Design review of the part built by this model. Coordinates are the model's own, in mm. A direction names the side the tool comes from. Coordinates: 2 decimals unless noted, no trailing zeros. Order: outer loops, then holes, each group sorted by start corner. A loop starts at its lowest first (then second) coordinate and runs counter-clockwise, first axis right, second up. Notation, with made-up numbers: M 65.25,-35.75 L 78.25,-35.75 A31 ccw 78.25,-7.75 Z; hole C 81,84.5 d7. An arc over 180 degrees is marked long. Use CSV: the item, a comma, the result in double quotes.
```python
from build123d import *

# Parameters (mm, degrees)
F0_W      = 63.5
F0_H      = 38.1
F1_DEPTH  = 38.1
F3_DEPTH  = 31.75
F4_R      = 6.35
F5_DEPTH  = 44.45
F6_R      = 3.175
F7_DEPTH  = 25.4
F9_DEPTH  = 25.4
F11_DEPTH = 25.4


# Not quite as in the source:
# - a length typed as a fraction of an inch, garbled in the dataset ("3 / 203.2 mm" for 3/8 in), is restored


with BuildPart() as f1:
    # F0 (on Top) → F1 (new body)
    with BuildSketch(Plane.XY):
        with Locations((-10.9044740348, 19.05)):
            Rectangle(F0_W, F0_H)
    extrude(amount=F1_DEPTH)

    # F2 (on face) → F3 (cut)
    with BuildSketch(Plane.XY.offset(38.1)):
        Polygon((-4.5544740348, 25.4), (-42.6544740348, 25.4), (-42.6544740348, 0), (20.8455259652, 0), (20.8455259652, 38.1), (-4.5544740348, 38.1), align=None)
    extrude(amount=-F3_DEPTH, mode=Mode.SUBTRACT)

    # F4 (on face) → F5 (cut)
    with BuildSketch(Plane.XZ.offset(-25.4)):
        with Locations((-29.9544740348, 25.4)):
            Circle(F4_R)
        with BuildLine():
            ThreePointArc((-42.6544740348, 25.4), (-38.9347301559, 34.3802561211), (-29.9544740348, 38.1))
            Line((-29.9544740348, 38.1), (-42.6544740348, 38.1))
            Line((-42.6544740348, 38.1), (-42.6544740348, 25.4))
        make_face()
        with BuildLine():
            ThreePointArc((-29.9544740348, 38.1), (-20.9742179137, 34.3802561211), (-17.2544740348, 25.4))
            ThreePointArc((-17.2544740348, 25.4), (-14.2002037714, 13.6778468423), (-4.5544740348, 6.35))
            Line((-4.5544740348, 6.35), (-4.5544740348, 38.1))
            Line((-4.5544740348, 38.1), (-29.9544740348, 38.1))
        make_face()
    extrude(amount=-F5_DEPTH, mode=Mode.SUBTRACT)

    # F6 (on face) → F7 (cut)
    with BuildSketch(Plane.XY.offset(6.35)):
        with Locations((11.3205259652, 9.525)):
            Circle(F6_R)
        with Locations((-33.1294740348, 9.525)):
            Circle(F6_R)
        with Locations((11.3205259652, 28.575)):
            Circle(F6_R)
    extrude(amount=-F7_DEPTH, mode=Mode.SUBTRACT)

    # F8 (on face) → F9 (cut)
    with BuildSketch(Plane.XY.offset(6.35)):
        with BuildLine():
            ThreePointArc((-36.3044740348, 0), (-40.7946020953, 1.8598719395), (-42.6544740348, 6.35))
            Line((-42.6544740348, 6.35), (-42.6544740348, 0))
            Line((-42.6544740348, 0), (-36.3044740348, 0))
        make_face()
    extrude(amount=-F9_DEPTH, mode=Mode.SUBTRACT)

    # F10 (on face) → F11 (cut)
    with BuildSketch(Plane.XY.offset(6.35)):
        with BuildLine():
            Line((20.8455259652, 0), (20.8455259652, 6.35))
            ThreePointArc((20.8455259652, 6.35), (18.9856540257, 1.8598719395), (14.4955259652, 0))
            Line((14.4955259652, 0), (20.8455259652, 0))
        make_face()
    extrude(amount=-F11_DEPTH, mode=Mode.SUBTRACT)


solid = f1.part
```
(1) Clearance check with flat-ended pins moving along their axes: P1, Ø5, axis at y = 31.5, z = 25, coming from the +X side; P2, Ø2, axis at x = -17, y = 10, coming from the +Z side; P3, Ø1, axis at x = -24, z = 33.5, coming from the -Y side. State where each tip first meets the part, or that it passes through.
The answers:
P1,"stops at x = -17.25"
P2,"stops at z = 6.35"
P3,"stops at y = 25.4"
(2) Add section C-C on x = -6. State the section outline as (y, z) points.
The answers:
outline,"M 0,0 L 38.1,0 L 38.1,6.89 L 25.4,6.89 L 25.4,6.35 L 0,6.35 Z"
(3) Add section D-D on z = 32.5. State the section outline as (x, y) points.
The answers:
outline,"M -40.48,25.4 L -19.42,25.4 L -19.42,38.1 L -40.48,38.1 Z"
(4) Add section B-B on y = 19.5. State the section outline as (x, z) points.
The answers:
outline,"M -42.65,0 L 20.85,0 L 20.85,6.35 L -42.65,6.35 Z"
(5) Wall thickness on probe 1 along Y at (x, z) = (-40, 11); probe 2 along Z at (x, y) = (-3, 19); probe 3 along X at (y, z) = (30, 28.5): over which ranges is each line inside the solid? List them lowest first.
The answers:
probe 1,"y = 25.4 to 38.1"
probe 2,"z = 0 to 6.35"
probe 3,"x = -42.27 to -35.5, -24.41 to -17.64"
(6) The part is to be moulded in two halves that separate along Z. For faces 1 (the face through (-36.3, 31.66, 25.68)), 2 (the face through (-42.654, 29, 10)), 3 (the face through (-11, 19, 0)), say which applies: pulls with the +Z half, pulls with the -Z half, needs draft (parallel to the pull), parting line crosses it, or undercut.
The answers:
face 1,"undercut"
face 2,"needs draft"
face 3,"pulls with the -Z half"
(7) For faces 4 (the face through (-28, 25.4, 19)), 5 (the face through (-11, 15, 6.35)), 6 (the face through (-18, 38.1, 15)), list the 3-axis set-ups (+Z, -Z, +X, -X, +Y, -Y) from which the entire face can be reached by the end or side of a thin tool; tool diameter is ignored.
The answers:
face 4,"+Z, +X, -X, -Y"
face 5,"+Z, +X, -Y"
face 6,"+Z, -Z, +X, -X, +Y"
(8) Add section A-A on x = -33.5. State the section outline as (y, z) points, and give its area (3 significant figures).
The answers:
outline,"M 0,0 L 6.37,0 L 6.37,6.35 L 0,6.35 Z; M 12.68,0 L 38.1,0 L 38.1,20.13 L 25.4,20.13 L 25.4,6.35 L 12.68,6.35 Z; M 25.4,30.67 L 38.1,30.67 L 38.1,37.6 L 25.4,37.6 Z"
area,"465 mm2"
